from build123d import *

# Parameters (mm, degrees)
F0_W     = 50
F0_H     = 100
F1_DEPTH = 1100
F2_W     = 100
F2_H     = 20
F3_DEPTH = 50.001
F5_DEPTH = 50.001


with BuildPart() as f1:
    # F0 (on Front) → F1 (new body)
    with BuildSketch(Plane.XZ):
        with Locations((25, 50)):
            Rectangle(F0_W, F0_H)
    extrude(amount=F1_DEPTH)

    # F2 (on face) → F3 (cut, through all)
    with BuildSketch(Plane.YZ.offset(50)):
        with Locations((-50, 10)):
            Rectangle(F2_W, F2_H)
        with Locations((-950, 10)):
            Rectangle(F2_W, F2_H)
    extrude(amount=-F3_DEPTH, mode=Mode.SUBTRACT)

    # F4 (on face) → F5 (cut, through all)
    with BuildSketch(Plane.YZ.offset(50)):
        with BuildLine():
            Line((-1030, 100), (-1070, 100))
            ThreePointArc((-1070, 100), (-1050, 80), (-1030, 100))
        make_face()
    extrude(amount=-F5_DEPTH, mode=Mode.SUBTRACT)


solid = f1.part
Geometry check sheet. Reference: the model listing, model coordinates, mm. A direction names the side the tool comes from. Round coordinates to 2 decimals unless told otherwise and drop trailing zeros. Order: outer loops, then holes, each group sorted by start corner. A loop starts at its lowest first (then second) coordinate and runs counter-clockwise, first axis right, second up. Notation, with made-up numbers: M -24.75,-32.5 L -7.75,-32.5 A25 ccw -7.75,0.5 Z; hole C 24,26 d9. An arc over 180 degrees is marked long. Answer in a Markdown table with one row per item.
(1) Tool access check on faces 1 (the face through (25, -1050, 80)), 2 (the face through (25, -100, 10)), 3 (the face through (25, -900, 10)). Record the directions out of +Z, -Z, +X, -X, +Y, -Y that give a thin tool (end or side, any length) a straight path to the whole face; none if there is none.
Responses:
| item | result |
|---|---|
| face 1 | +Z, +X, -X |
| face 2 | -Z, +X, -X, +Y |
| face 3 | -Z, +X, -X |
(2) Sectioned sample at B-B, the plane y = -1050. Record the cut outline in (x, z), and give its area (3 significant figures).
Responses:
| item | result |
|---|---|
| outline | M 0,0 L 50,0 L 50,80 L 0,80 Z |
| area | 4,000 mm² |
(3) Go/stop test with flat-tipped pins: P1, Ø25, axis at x = 19.5, y = -26.5, coming from the -Z side; P2, Ø16, axis at x = 31.5, z = 13, coming from the +Y side; P3, Ø6, axis at x = 14.5, z = 11.5, coming from the +Y side. Record where each tip stops, or that it passes through.
Responses:
| item | result |
|---|---|
| P1 | stops at z = 20 |
| P2 | stops at y = 0 |
| P3 | stops at y = -100 |
(4) Sectioned sample at A-A, the plane x = 12. Record the cut outline in (y, z), and give its area (3 significant figures).
Responses:
| item | result |
|---|---|
| outline | M -1100,0 L -1000,0 L -1000,20 L -900,20 L -900,0 L -100,0 L -100,20 L 0,20 L 0,100 L -1030,100 A20 cw -1070,100 L -1100,100 Z |
| area | 105,000 mm² |
(5) Scan lines: probe 1 along Y at (x, z) = (45.5, 16); probe 2 along Z at (x, y) = (13, -1049.5); probe 3 along Y at (x, z) = (28.5, 84). Record each from-to range of solid material in increasing order. Write a range as from..to.
Responses:
| item | result |
|---|---|
| probe 1 | y = -1100..-1000, -900..-100 |
| probe 2 | z = 0..80.01 |
| probe 3 | y = -1100..-1062, -1038..0 |
